Model file for the job. Use its own axes, mm. A direction names the side the tool comes from. Coordinates: 2 decimals unless noted, no trailing zeros. Write each loop counter-clockwise with the first axis right and the second up, starting at its lowest first coordinate (ties: lowest second). Pieces come first, ordered by that corner, then holes. Notation, with made-up numbers: (-13.5, -13.75) - (-1.5, -13.75) arc R28 ccw to (-1.5, 7.25) - close; hole circle Ø10 at (89.5, -33.75). An arc over 180 degrees is marked (long way). Put each result on its own line as item: value. Start each with the question number.
1. Which spindle directions (+Z, -Z, +X, -X, +Y, -Y) get a long thin tool onto all of the face, cutting with end or side? Do faces 1 (the face through (1, -36, 9.525)), 2 (the face through (34.95, 16.55, 49.7)), 3 (the face through (48, -25.4, 45)), 4 (the face through (45.8, -0.4, 38.1)). Say none if no direction does.
2. Saw through at A-A, the plane y = -48. Write the cut outline in (x, z) (3 decimals), plus the area to 3 significant figures.
3. Saw through at C-C, the plane y = 14. Write the cut outline in (x, z) (3 decimals).
4. Drill centre lines: L1, parallel to X at y = -41, z = -3.5 (3 decimals); L2, parallel to Z at x = 59, y = -20.5; L3, parallel to Y at x = 30, z = 17. Where is each one in solid material? Low to high. Write a range as from..to.
5. Saw through at D-D, the plane y = -11.5. Write the cut outline in (x, z) (3 decimals), plus the area to 3 significant figures.
6. Drop flat-ended pins along their axis: P1, Ø5, axis at y = -16.5, z = 15, coming from the -X side; P2, Ø5, axis at x = 60, z = 49.5, coming from the -Y side; P3, Ø12, axis at x = 59, y = -5, coming from the +Z side (3 decimals); P4, Ø2, axis at y = -3.5, z = 15, coming from the -X side. Give the stop position or say it passes through.
7. Saw through at B-B, the plane x = 100. Write the cut outline in (y, z) (3 decimals).
```python
from build123d import *

# Parameters (mm, degrees)
F1_DEPTH = 63.5
F2_DEPTH = 7.9375
F3_DEPTH = 25.4
F4_DEPTH = 25.4
F6_R     = 6.35


with BuildPart() as f1:
    # F0 (on Front) → F1 (new body, symmetric)
    with BuildSketch(Plane.XZ):
        Polygon((-41.275, 9.525), (-41.275, -9.525), (41.275, -9.525), (41.275, 9.525), (25.4, 9.525), align=None)
    extrude(amount=F1_DEPTH, both=True)

    # F0 (on Front) → F2 (join, symmetric)
    with BuildSketch(Plane.XZ):
        with BuildLine():
            add(Edge.make_bspline(
                [(-41.275, 9.525), (-37.399922, 44.91622), (23.305045, 59.918404), (60.325, 58.7502)],
                knots=[0, 0, 0, 0, 112.896768, 112.896768, 112.896768, 112.896768], degree=3))
            Line((-41.275, 9.525), (25.4, 9.525))
            Line((25.4, 9.525), (25.4, 27.0002))
            ThreePointArc((25.4, 27.0002), (34.69936, 49.45084), (57.15, 58.7502))
            Line((57.15, 58.7502), (60.325, 58.7502))
        make_face()
    extrude(amount=F2_DEPTH, both=True)

    # F0 (on Front) → F3 (join, symmetric)
    with BuildSketch(Plane.XZ):
        with BuildLine():
            Line((25.4, 9.525), (41.275, 9.525))
            Line((41.275, 9.525), (41.275, 27.0002))
            ThreePointArc((41.275, 27.0002), (45.92468, 38.22552), (57.15, 42.8752))
            Line((57.15, 42.8752), (60.325, 42.8752))
            Line((60.325, 42.8752), (60.325, 58.7502))
            Line((60.325, 58.7502), (57.15, 58.7502))
            ThreePointArc((57.15, 58.7502), (34.69936, 49.45084), (25.4, 27.0002))
            Line((25.4, 27.0002), (25.4, 9.525))
        make_face()
    extrude(amount=F3_DEPTH, both=True)

    # F0 (on Front) → F4 (join, symmetric)
    with BuildSketch(Plane.XZ):
        Polygon((80.22992, 58.7502), (60.325, 58.7502), (60.325, 42.8752), (80.22992, 42.8752), (85.725, 42.8752), (85.725, 58.7502), align=None)
    extrude(amount=F4_DEPTH, both=True)

    # F0 (on Front) → F5 (revolve)
    with BuildSketch(Plane.XZ):
        Polygon((111.125, 66.675), (85.725, 66.675), (85.725, 58.7502), (85.725, 42.8752), (85.725, 38.1), (111.125, 38.1), align=None)
    revolve(axis=Axis((85.725, 0, 52.3875), (0, 0, 1)))

    # F6
    f6_edges = [f1.edges().sort_by_distance(p)[0] for p in [
        (41.275, -63.5, 0),
        (-41.275, -63.5, 0),
        (41.275, 63.5, 0),
        (-41.275, 63.5, 0),
    ]]
    fillet(f6_edges, radius=F6_R)


solid = f1.part
```
Final values:
1. face 1: +Z, -X, -Y
1. face 2: +Z, -X, +Y
1. face 3: +Z, +X, -X, -Y
1. face 4: -Z, +Y, -Y
2. outline: (-41.275, -9.525) - (41.275, -9.525) - (41.275, 9.525) - (-41.275, 9.525) - close
2. area: 1,570 mm²
3. outline: (-41.275, -9.525) - (41.275, -9.525) - (41.275, 27) arc R15.875 cw to (57.15, 42.875) - (64.532, 42.875) - (64.532, 38.1) - (106.918, 38.1) - (106.918, 66.675) - (64.532, 66.675) - (64.532, 58.75) - (57.15, 58.75) arc R31.75 ccw to (25.4, 27) - (25.4, 9.525) - (-41.275, 9.525) - close
4. L1: x = -41.275..41.275
4. L2: z = 42.88..58.75
4. L3: y = -25.4..25.4
5. outline: (-41.275, -9.525) - (41.275, -9.525) - (41.275, 27) arc R15.875 cw to (57.15, 42.875) - (63.077, 42.875) - (63.077, 38.1) - (108.373, 38.1) - (108.373, 66.675) - (63.077, 66.675) - (63.077, 58.75) - (57.15, 58.75) arc R31.75 ccw to (25.4, 27) - (25.4, 9.525) - (-41.275, 9.525) - close
5. area: 3,830 mm²
6. P1: stops at x = 25.4
6. P2: stops at y = -25.4
6. P3: stops at z = 66.675
6. P4: stops at x = -40.46
7. outline: (-21.009, 38.1) - (21.009, 38.1) - (21.009, 66.675) - (-21.009, 66.675) - close
